Could you check a few things on this model? Use its own coordinates, in mm. A direction names the side the tool comes from. Give positions to 0.01 mm unless a question says otherwise; leave off trailing zeros. Order: outer loops, then holes, each group sorted by start corner. A loop starts at its lowest first (then second) coordinate and runs counter-clockwise, first axis right, second up. Notation, with made-up numbers: M -2.75,23 L 43.25,23 A28 ccw 43.25,43 Z; hole C -16,12.25 d10. An arc over 180 degrees is marked long. Use a Markdown table: item, result. Add a question column.
Item 1: For faces 1 (the face through (12, -15, 28)), 2 (the face through (12, 0, 13)), 3 (the face through (8, -15, -3)), which set-ups out of +Z, -Z, +X, -X, +Y, -Y let a thin tool reach every point of the face, with its end or its side?
Item 2: Suppose I cut it at A-A on x = 14.25. Write out the boundary of the cut face in (y, z), plus the area to 3 significant figures.
Item 3: If I drill on L1, parallel to Y at x = 3.5, z = -5; L2, parallel to Z at x = 15, y = -29; L3, parallel to Z at x = 17, y = -9, over which ranges is the centre line in solid material (lowest first)? Write a range as from..to.
Item 4: Suppose I cut it at B-B on y = -5. Write out the boundary of the cut face in (x, z).
Item 5: I'm going to push flat-ended pins straight in: pin 1 Ø12 at (x, y) = (3, -25.5) entering from -Z; pin 2 Ø12 at (x, y) = (12.5, -37.5) entering from +Z; pin 3 Ø2 at (x, y) = (11.5, -7.5) entering from -Z. Where does each tip first touch, or does it pass through?
Item 6: Suppose I cut it at C-C on z = 26.5. Write out the boundary of the cut face in (x, y).
Item 7: Suppose I cut it at D-D on x = 21.5. Write out the boundary of the cut face in (y, z), plus the area to 3 significant figures.
from build123d import *

# Parameters (mm, degrees)
F0_W     = 24.481318
F0_H     = 25
F1_DEPTH = 63.5
F2_R     = 7.5
F3_DEPTH = 15
F4_R     = 7.5
F5_DEPTH = 15


with BuildPart() as f1:
    # F0 (on Front) → F1 (new body)
    with BuildSketch(Plane.XZ):
        with Locations((12.240659, 12.5)):
            Rectangle(F0_W, F0_H)
    extrude(amount=F1_DEPTH)

    # F2 (on Front) → F3 (join)
    with BuildSketch(Plane.XZ):
        with Locations((12.228578, 25.193848)):
            Circle(F2_R)
    extrude(amount=F3_DEPTH)

    # F4 (on Front) → F5 (join)
    with BuildSketch(Plane.XZ):
        with Locations((8.243513, 0)):
            Circle(F4_R)
    extrude(amount=F5_DEPTH)


solid = f1.part
Findings below:
| question | item | result |
|---|---|---|
| 1 | face 1 | +Z, +X, -X, -Y |
| 1 | face 2 | +Z, -Z, +X, -X, +Y |
| 1 | face 3 | -Z, +X, -X, -Y |
| 2 | outline | M -63.5,0 L -15,0 L -15,-4.49 L 0,-4.49 L 0,32.42 L -15,32.42 L -15,25 L -63.5,25 Z |
| 2 | area | 1,770 mm^2 |
| 3 | L1 | y = -15..0 |
| 3 | L2 | z = 0..25 |
| 3 | L3 | z = 0..30.98 |
| 4 | outline | M 0,0 L 0.74,0 A7.5 ccw 15.74,0 L 24.48,0 L 24.48,25 L 19.73,25 A7.5 ccw long 4.73,25 L 0,25 Z |
| 5 | pin 1 | stops at z = 0 |
| 5 | pin 2 | stops at z = 25 |
| 5 | pin 3 | stops at z = -7.15 |
| 6 | outline | M 4.84,-15 L 19.61,-15 L 19.61,0 L 4.84,0 Z |
| 7 | outline | M -63.5,0 L 0,0 L 0,25 L -63.5,25 Z |
| 7 | area | 1,590 mm^2 |
